```python
from build123d import *

# Parameters (mm, degrees)
F0_R     = 6.35
F1_DEPTH = 46.736
F2_R     = 10.795
F2_R_2   = 4
F3_DEPTH = 12.7
F4_R     = 3.81
F5_DEPTH = 7.62


with BuildPart() as f1:
    # F0 (on Front) → F1 (new body)
    with BuildSketch(Plane.XZ):
        Circle(F0_R)
    extrude(amount=F1_DEPTH)

    # F2 (on Front) → F3 (join)
    with BuildSketch(Plane.XZ):
        Circle(F2_R)
        Circle(F2_R_2, mode=Mode.SUBTRACT)
    extrude(amount=-F3_DEPTH)

    # F4 (on face) → F5 (cut)
    with BuildSketch(Plane.XZ.offset(46.736)):
        Circle(F4_R)
    extrude(amount=-F5_DEPTH, mode=Mode.SUBTRACT)


solid = f1.part
```
Work out the finished part from the listing and answer in its coordinate system (mm). A direction names the side the tool comes from. Give positions to 0.01 mm unless a question says otherwise; leave off trailing zeros. Loops run counter-clockwise (first coordinate to the right, second up) from the corner with the lowest first, then second, coordinate; pieces in that order, holes last. Notation, with made-up numbers: (54, 62) -> (98, 62) arc R19 ccw to (98, 67) -> close; hole circle Ø1 at (24.25, 40.5). An arc over 180 degrees is marked (long way). Put each result on its own line as item: value. Start each with the question number.
Item 1: Which of the six approach directions +Z, -Z, +X, -X, +Y, -Y give full straight-line access (tool end or side, diameter ignored) to faces 4 (the face through (0, -39.116, 0)), 5 (the face through (5, 12.7, 0)), 6 (the face through (-0.867, 6.261, -3.905))?
Item 2: The mould has two halves that part along X. Classify faces 1 (the face through (5, 0, -5)), 2 (the face through (-1.38, -23.04, -6.2)), 3 (the face through (-0.83, -42.98, -3.72)): released by +X, released by -X, zero draft, split by the parting line, or undercut.
Item 3: The part is cut by section D-D (y = -26.5). Give the vertices of the cut face in (x, z).
Item 4: The part is cut by section B-B (y = -41). Give the vertices of the cut face in (x, z), then the cut area to 3 significant figures.
Item 5: The part is cut by section C-C (z = 0). Give the vertices of the cut face in (x, y) (3 decimals).
Item 6: The part is cut by section A-A (x = 0). Give the vertices of the cut face in (y, z) (3 decimals), then the cut area to 3 significant figures.
Item 7: Each of these flat-tipped pins is pushed along its axis until it touches: P1, Ø2.5, axis at x = 0, z = -0.5, coming from the -Y side; P2, Ø3, axis at x = 8.5, z = 7, coming from the +Y side; P3, Ø12, axis at x = -6, y = -23.5, coming from the -Z side; P4, Ø4, axis at x = 5, y = 1.5, coming from the -Z side. Where does it stop, or does it pass through?
Item 8: Find the intervals of material crossed by L1, parallel to Z at x = 0, y = 5.75 (3 decimals); L2, parallel to Z at x = 0, y = -41; L3, parallel to Y at x = 7.5, z = -7.5, in increasing order. Write a range as [from, to].
Answers below:
1. face 4: -Y
1. face 5: +Z, -Z, +X, -X, +Y
1. face 6: +Y
2. face 1: zero draft
2. face 2: split by the parting line
2. face 3: undercut
3. outline: circle Ø12.7 at (0, 0)
4. outline: circle Ø12.7 at (0, 0); hole circle Ø7.62 at (0, 0)
4. area: 81.1 mm2
5. outline: (-10.795, 0) -> (-6.35, 0) -> (-6.35, -46.736) -> (-3.81, -46.736) -> (-3.81, -39.116) -> (3.81, -39.116) -> (3.81, -46.736) -> (6.35, -46.736) -> (6.35, 0) -> (10.795, 0) -> (10.795, 12.7) -> (4, 12.7) -> (4, 0) -> (-4, 0) -> (-4, 12.7) -> (-10.795, 12.7) -> close
6. outline: (-46.736, -6.35) -> (0, -6.35) -> (0, -10.795) -> (12.7, -10.795) -> (12.7, -4) -> (0, -4) -> (0, 4) -> (12.7, 4) -> (12.7, 10.795) -> (0, 10.795) -> (0, 6.35) -> (-46.736, 6.35) -> (-46.736, 3.81) -> (-39.116, 3.81) -> (-39.116, -3.81) -> (-46.736, -3.81) -> close
6. area: 708 mm2
7. P1: y = -39.12
7. P2: y = 12.7
7. P3: z = -6.35
7. P4: z = -10.37
8. L1: [-10.795, -4], [4, 10.795]
8. L2: [-6.35, -3.81], [3.81, 6.35]
8. L3: [0, 12.7]
